Check sheet for the drawn part. Datum: minimum x, y, z corner. Units: mm. A direction names the side the tool comes from. Round coordinates to 2 decimals unless told otherwise and drop trailing zeros. Write each loop counter-clockwise with the first axis right and the second up, starting at its lowest first coordinate (ties: lowest second). Pieces come first, ordered by that corner, then holes. Notation, with made-up numbers: (35, 0) - (82, 0) arc R8 ccw to (82, 10) - close; hole circle Ø7 at (43, 39.5). An arc over 180 degrees is marked (long way). Answer as a JSON object with one key per item and string values.
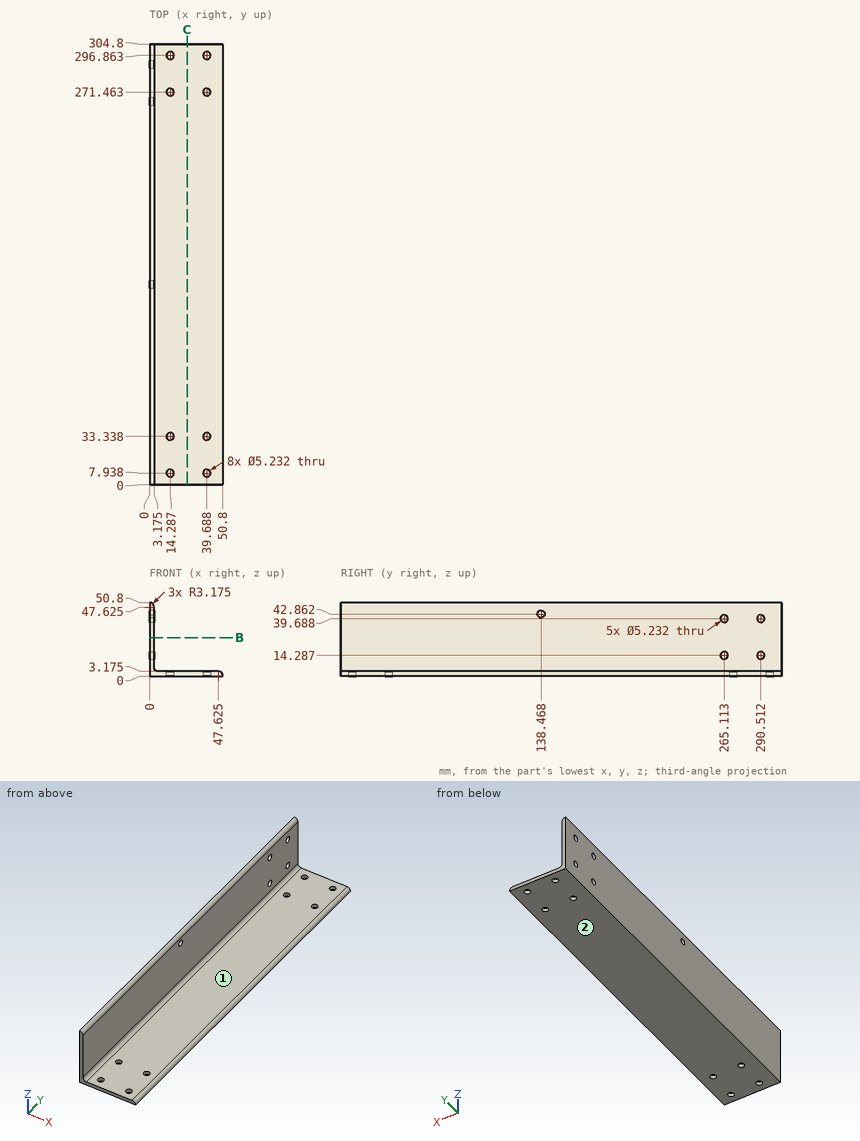
1. Cross-section at C-C (x = 26). Record the boundary of the cut face in (y, z) (1 decimal).
Completed:
{"outline": "(0, 0) - (304.8, 0) - (304.8, 3.2) - (0, 3.2) - close"}
2. Go/stop test with flat-tipped pins: pin 1 (3 mm diameter, centred on x = 39.69, y = 7.94, fed in from -Z); pin 2 (5 mm diameter, centred on y = 137, z = 32.5, fed in from +X) (1 decimal); pin 3 (8.5 mm diameter, centred on x = 39.69, y = 33.34, fed in from +Z) (1 decimal). Record where each tip stops, or that it passes through.
Completed:
{"pin 1": "passes through", "pin 2": "stops at x = 3.2", "pin 3": "stops at z = 3.2"}
3. Access from +Z, -Z, +X, -X, +Y, -Y to the whole of each face (thin tool, end or side, straight path). Record for the marked faces 1 and 2.
Completed:
{"face 1": "+Z, +X, +Y, -Y", "face 2": "-Z, +X, -X, +Y, -Y"}
4. Material ranges on probe 1 along Y at (x, z) = (3, 12.5) (1 decimal); probe 2 along X at (y, z) = (113.5, 22) (1 decimal), recorded low to high. Write a range as from..to.
Completed:
{"probe 1": "y = 0..263.2, 267..288.6, 292.4..304.8", "probe 2": "x = 0..3.2"}
5. Cross-section at B-B (z = 26.5). Record the boundary of the cut face in (x, y) (1 decimal).
Completed:
{"outline": "(0, 0) - (3.2, 0) - (3.2, 304.8) - (0, 304.8) - close"}
